```python
from build123d import *

# Parameters (mm, degrees)
SKETCH_1_R                    = 50
EXTRUDE_1_DEPTH               = 10
HOLE_WIZARD_M10_1_D           = 8.5
HOLE_WIZARD_M10_1_CSINK_D     = 10.05
HOLE_WIZARD_M10_1_CSINK_ANGLE = 90
SKETCH_16_W                   = 65
SKETCH_16_H                   = 10
EXTRUDE_2_DEPTH               = 30
SKETCH_18_W                   = 65
SKETCH_18_H                   = 8.750492466
EXTRUDE_3_DEPTH               = 40
FILLET_2_R                    = 10
FILLET_3_R                    = 10
CUT_EXTRUDE_1_REACH           = 104.364
SKETCH_20_R                   = 2.5
CUT_EXTRUDE_2_REACH           = 100.203
SKETCH_22_R                   = 6


with BuildPart() as part:
    # 草图1 → 凸台-拉伸1 (new body)
    with BuildSketch(Plane.XY):
        Circle(SKETCH_1_R)
    extrude(amount=EXTRUDE_1_DEPTH)

    # M10 螺纹孔1 (through all)
    with Locations(Plane.XY.offset(10)):
        with Locations((-20.426671729, 0)):
            hole_wizard_m10_1 = CounterSinkHole(HOLE_WIZARD_M10_1_D / 2, HOLE_WIZARD_M10_1_CSINK_D / 2, counter_sink_angle=HOLE_WIZARD_M10_1_CSINK_ANGLE)

    # 镜向2: M10 螺纹孔1 across plane
    add(hole_wizard_m10_1.mirror(Plane(origin=(0, 0, 0), x_dir=(0, 0, 1), z_dir=(1, 0, 0))), mode=Mode.SUBTRACT)

    # 草图16 → 凸台-拉伸2 (add)
    with BuildSketch(Plane.XY.offset(10)):
        with Locations((0, -24.864937428)):
            Rectangle(SKETCH_16_W, SKETCH_16_H)
    extrude(amount=EXTRUDE_2_DEPTH)

    # 草图18 → 凸台-拉伸3 (add)
    with BuildSketch(Plane.XY.offset(10)):
        with Locations((0, 20.081420938)):
            Rectangle(SKETCH_18_W, SKETCH_18_H)
    extrude(amount=-EXTRUDE_3_DEPTH)

    # 圆角2
    fillet_2_edges = [part.edges().sort_by_distance(p)[0] for p in [
        (-32.5, -24.864937428, 40),
        (32.5, -24.864937428, 40),
    ]]
    fillet(fillet_2_edges, radius=FILLET_2_R)

    # 圆角3
    fillet_3_edges = [part.edges().sort_by_distance(p)[0] for p in [
        (32.5, 20.081420938, -30),
        (-32.5, 20.081420938, -30),
    ]]
    fillet(fillet_3_edges, radius=FILLET_3_R)

    # 草图20 → 切除-拉伸1 (cut, up to next)
    with BuildSketch(Plane.XZ.offset(29.864937428), mode=Mode.PRIVATE) as cut_extrude_1_sk1:
        with Locations(Location((-15, 28, 0), (0, 0, 270))):
            Circle(SKETCH_20_R)
    cut_extrude_1_tool1 = extrude(cut_extrude_1_sk1.sketch, amount=-CUT_EXTRUDE_1_REACH, mode=Mode.PRIVATE) & part.part
    # 草图20 → 切除-拉伸1 (cut, up to next)
    with BuildSketch(Plane.XZ.offset(29.864937428), mode=Mode.PRIVATE) as cut_extrude_1_sk2:
        with Locations(Location((15, 28, 0), (0, 0, 90))):
            Circle(SKETCH_20_R)
    cut_extrude_1_tool2 = extrude(cut_extrude_1_sk2.sketch, amount=-CUT_EXTRUDE_1_REACH, mode=Mode.PRIVATE) & part.part
    add(cut_extrude_1_tool1.solids().sort_by_distance((-15, -29.864937, 28))[0], mode=Mode.SUBTRACT)
    add(cut_extrude_1_tool2.solids().sort_by_distance((15, -29.864937, 28))[0], mode=Mode.SUBTRACT)

    # 草图22 → 切除-拉伸2 (cut, up to next)
    with BuildSketch(Plane(origin=(0, 24.456667171, 0), x_dir=(1, 0, 0), z_dir=(0, 1, 0)), mode=Mode.PRIVATE) as cut_extrude_2_sk1:
        with Locations(Location((-15, 14.615729017, 0), (0, 0, 270))):
            Circle(SKETCH_22_R)
    cut_extrude_2_tool1 = extrude(cut_extrude_2_sk1.sketch, amount=-CUT_EXTRUDE_2_REACH, mode=Mode.PRIVATE) & part.part
    # 草图22 → 切除-拉伸2 (cut, up to next)
    with BuildSketch(Plane(origin=(0, 24.456667171, 0), x_dir=(1, 0, 0), z_dir=(0, 1, 0)), mode=Mode.PRIVATE) as cut_extrude_2_sk2:
        with Locations(Location((15, 14.615729017, 0), (0, 0, 90))):
            Circle(SKETCH_22_R)
    cut_extrude_2_tool2 = extrude(cut_extrude_2_sk2.sketch, amount=-CUT_EXTRUDE_2_REACH, mode=Mode.PRIVATE) & part.part
    add(cut_extrude_2_tool1.solids().sort_by_distance((-15, 24.456667, -14.615729))[0], mode=Mode.SUBTRACT)
    add(cut_extrude_2_tool2.solids().sort_by_distance((15, 24.456667, -14.615729))[0], mode=Mode.SUBTRACT)


solid = part.part
```
The model under review builds one solid part; all positions refer to its coordinate system, in mm. A direction names the side the tool comes from. Give positions to 0.01 mm unless a question says otherwise; leave off trailing zeros. Write each loop counter-clockwise with the first axis right and the second up, starting at its lowest first coordinate (ties: lowest second). Pieces come first, ordered by that corner, then holes. Notation, with made-up numbers: (65.25, 11.5) - (99.25, 11.5) arc R16 ccw to (99.25, 29.5) - close; hole circle Ø1 at (18.5, 26). An arc over 180 degrees is marked (long way). Answer in a Markdown table with one row per item. Add a question column.
1. Insertion check: P1, Ø9, axis at x = -6, z = 22.5, coming from the +Y side; P2, Ø12, axis at x = -13, z = 7, coming from the +Y side; P3, Ø4.5, axis at y = 22, z = -9.5, coming from the +X side; P4, Ø3, axis at x = 15, z = 28, coming from the +Y side. Each pin has a flat end and moves straight along its axis. Give the tip position at first contact, or say it passes through.
2. Wall thickness on line 1 along X through (y, z) = (-22, 28); line 2 along Z through (x, y) = (13.5, -34); line 3 along Y through (x, z) = (-14, -2): over which ranges is each line inside the solid? List them lowest first. Write a range as [from, to].
3. We need section A-A on y = 0. Write out the cut boundary in (x, z) (3 decimals).
4. We need section C-C on x = 0. Write out the cut boundary in (y, z).
5. Tool access review of faces 1 (the flat face through (-32.5, -25, 20)), 2 (the flat face through (0, 15.706, -15)), 3 (the flat face through (32.5, 20, -10)), 4 (the flat face through (-32.5, 20, -10)), 5 (the cylindrical face through (16.5, -24.9, 26)): name each direction out of +Z, -Z, +X, -X, +Y, -Y from which nothing blocks a thin tool from reaching the whole face with its end or side.
6. Draft analysis for pull direction Y (two halves, no side actions). For faces 6 (the cylindrical face through (16.18, 0.19, 4.55)), 7 (the cylindrical face through (29.65, -24.79, 36.99)), 8 (the flat face through (0, -19.865, 25)), state which applies: +Y half, -Y half, draft (parallel to the pull), parting line (faces both ways), or undercut.
7. We need section B-B on z = 28. Write out the cut boundary in (x, y).
8. We need section D-D on y = 18. Write out the cut boundary in (x, z).
Ans:
| question | item | result |
|---|---|---|
| 1 | P1 | stops at y = -19.86 |
| 1 | P2 | stops at y = 49.51 |
| 1 | P3 | stops at x = 32.5 |
| 1 | P4 | passes through |
| 2 | line 1 | x = [-32.5, -17.5], [-12.5, 12.5], [17.5, 32.5] |
| 2 | line 2 | z = [0, 10] |
| 2 | line 3 | y = [15.71, 24.46] |
| 3 | outline | (-50, 0) - (-24.677, 0) - (-24.677, 9.225) - (-25.452, 10) - (-50, 10) - close; (-16.177, 0) - (16.177, 0) - (16.177, 9.225) - (15.402, 10) - (-15.402, 10) - (-16.177, 9.225) - close; (24.677, 0) - (50, 0) - (50, 10) - (25.452, 10) - (24.677, 9.225) - close |
| 4 | outline | (-50, 0) - (15.71, 0) - (15.71, -30) - (24.46, -30) - (24.46, 0) - (50, 0) - (50, 10) - (-19.86, 10) - (-19.86, 40) - (-29.86, 40) - (-29.86, 10) - (-50, 10) - close |
| 5 | face 1 | +Z, -X, +Y, -Y |
| 5 | face 2 | -Z, +X, -X, -Y |
| 5 | face 3 | -Z, +X, +Y, -Y |
| 5 | face 4 | -Z, -X, +Y, -Y |
| 5 | face 5 | +Y, -Y |
| 6 | face 6 | undercut |
| 6 | face 7 | draft |
| 6 | face 8 | +Y half |
| 7 | outline | (-32.5, -29.86) - (-17.5, -29.86) - (-17.5, -19.86) - (-32.5, -19.86) - close; (-12.5, -29.86) - (12.5, -29.86) - (12.5, -19.86) - (-12.5, -19.86) - close; (17.5, -29.86) - (32.5, -29.86) - (32.5, -19.86) - (17.5, -19.86) - close |
| 8 | outline | (-46.65, 0) - (-32.5, 0) - (-32.5, -20) arc R10 ccw to (-22.5, -30) - (22.5, -30) arc R10 ccw to (32.5, -20) - (32.5, 0) - (46.65, 0) - (46.65, 10) - (-46.65, 10) - close; hole circle Ø12 at (-15, -14.62); hole circle Ø12 at (15, -14.62) |
